The model under review builds one solid part; all positions refer to its coordinate system, in mm. A direction names the side the tool comes from. Give positions to 0.01 mm unless a question says otherwise; leave off trailing zeros. Loops run counter-clockwise (first coordinate to the right, second up) from the corner with the lowest first, then second, coordinate; pieces in that order, holes last. Notation, with made-up numbers: M 26.5,-9 L 50.5,-9 A17 ccw 50.5,8 Z; hole C 78,8 d9. An arc over 180 degrees is marked long. Write item = value, one per line. Start each with the question number.
1. For faces 1 (the face through (5, 41, -19)), 2 (the face through (4, 41, -29.25)), 3 (the face through (6, 41, -31)), list the 3-axis set-ups (+Z, -Z, +X, -X, +Y, -Y) from which the entire face can be reached by the end or side of a thin tool; tool diameter is ignored.
2. We need section B-B on z = -34. Give the boundary of the cut face in (x, y), then the cut area to 3 significant figures.
3. Wall thickness on line 1 along Z through (x, y) = (2.35, 71); line 2 along Z through (x, y) = (5, 39); line 3 along Z through (x, y) = (2.25, 71): over which ranges is each line inside the solid? List them lowest first. Write a range as from..to.
4. We need section D-D on y = 67.5. Give the boundary of the cut face in (x, z).
5. Draft analysis for pull direction Y (two halves, no side actions). For faces 4 (the face through (1, 14, -17)), 5 (the face through (1.479, 72.908, -15.601)), 6 (the face through (3, 40, -39)), 7 (the face through (2, 0, -13)), state which applies: pulls with the +Y half, pulls with the -Y half, needs draft (parallel to the pull), parting line crosses it, or undercut.
6. For pin 1 (5.5 mm diameter, centred on x = 3.5, y = 55.5, fed in from +Z); pin 2 (4.5 mm diameter, centred on y = 71, z = -15, fed in from +X); pin 3 (5 mm diameter, centred on x = 10.5, y = 38.5, fed in from +Z); pin 4 (2.5 mm diameter, centred on y = 14, z = -15, fed in from +X), all flat-tipped, find the tip position at first contact; note any pin that passes through.
7. We need section A-A on y = 14. Count the separate pieces of the cut face and the enclosed holes in it, then the cut area to 3 significant figures.
8. We need section C-C on x = 6. Give the boundary of the cut face in (y, z), then the cut area to 4 significant figures.
Autodesk Inventor part; units mm, degrees
ref_plane "YZ Plane" through (0, 0, 0) normal (1, 0, 0) x (0, 1, 0)
ref_plane "XZ Plane" through (0, 0, 0) normal (0, 1, 0) x (-1, 0, 0)
ref_plane "XY Plane" through (0, 0, 0) normal (0, 0, 1) x (1, 0, 0)
sketch "Sketch1" plane through (0, 0, 0) normal (1, 0, 0) x (0, 1, 0)
  line L0 (0, 0) -> (81, 0)
  line L1 (81, 0) -> (81, -50)
  line L2 (81, -50) -> (0, -50)
  line L3 (0, -50) -> (0, 0)
  circle A0 centre (71, -15) radius 2
  circle A1 centre (71, -34) radius 2
  circle A2 centre (14, -15) radius 2
  circle A3 centre (14, -34) radius 2
  dimension "d0" = 81
  dimension "d1" = 50
  dimension "d2" = 4
  dimension "d3" = 15
  dimension "d4" = 4
  dimension "d5" = 16
  dimension "d6" = 4
  dimension "d7" = 15
  dimension "d8" = 4
  dimension "d9" = 57
  dimension "d11" = 10
  dimension "d12" = 57
  dimension "d13" = 10
extrude "Extrusion1" add sketch "Sketch1" along normal blind 3
sketch "Sketch5" plane through (0, 81, 0) normal (0, 1, 0) x (1, 0, 0)
  circle A0 centre (7, 25) radius 4
  line L0 (0, 0) -> (3, 0)
  line L1 (3, 50) -> (3, 0)
  dimension "d26" = 8
  dimension "d27" = 25
  dimension "d28" = 4
extrude "Extrusion3" add sketch "Sketch5" against normal blind 81
sketch "Sketch9" plane through (7, 81, -25) normal (0, 1, 0) x (1, 0, 0)
  line L0 (-4, 0) -> (-4, -25)
  line L1 (-4, -6) -> (6, -6)
  line L2 (6, -6) -> (6, 6)
  line L3 (6, 6) -> (-4, 6)
  line L4 (-4, 6) -> (-4, -6)
  line L5 (-7, -25) -> (-4, -25)
  dimension "d42" = 10
  dimension "d43" = 12
  dimension "d44" = 19
extrude "Extrusion6" add sketch "Sketch9" against normal blind 81
sketch "Sketch10" plane through (0, 81, 0) normal (0, 1, 0) x (1, 0, 0)
  line L0 (3, 19) -> (13, 19)
  line L1 (13, 19) -> (13, 31)
  line L2 (7, 29.25) -> (0, 29.25)
  line L3 (0, 50) -> (0, 0)
  line L4 (7, 20.75) -> (0, 20.75)
  arc A0 (7, 20.75) -> (7, 29.25) centre (7, 25) ccw
  arc A1 (7, 20.75) -> (7, 29.25) centre (7, 25) ccw
  arc A2 (7, 20.75) -> (7, 29.25) centre (7, 25) ccw
  dimension "d55" = 4.25
  dimension "d56" = 4.25
  dimension "d57" = 4.25
extrude "Extrusion8" cut sketch "Sketch10" against normal blind 81
fillet "Fillet4" radius 4 2 edges at (3, 40.5, 0) (3, 40.5, -50)
fillet "Fillet5" radius 1 2 edges at (3, 40.5, -19) (3, 40.5, -31)
fillet "Fillet6" radius 6 4 edges at (13, 81, -25) (13, 0, -25) (13, 40.5, -19) (13, 40.5, -31)
Final values:
q1.face_1 = +Z, +X, +Y, -Y
q1.face_2 = -X, +Y, -Y
q1.face_3 = -Z, +X, +Y, -Y
q2.outline = M 0,0 L 3,0 L 3,12 L 0,12 Z; M 0,16 L 3,16 L 3,69 L 0,69 Z; M 0,73 L 3,73 L 3,81 L 0,81 Z
q2.area = 219 mm²
q3.line_1 = -48.31..-36, -32..-29.25, -20.75..-17, -13..-1.69
q3.line_2 = -31..-29.25, -20.75..-19
q3.line_3 = -48.46..-36, -32..-29.25, -20.75..-17, -13..-1.54
q4.outline = M 0,-50 A4 ccw 3,-46.13 L 3,-32 A1 cw 4,-31 L 7,-31 A6 ccw 7,-19 L 4,-19 A1 cw 3,-18 L 3,-3.87 A4 ccw 0,0 L 0,-20.75 L 7,-20.75 A4.25 cw 7,-29.25 L 0,-29.25 Z
q5.face_4 = undercut
q5.face_5 = undercut
q5.face_6 = needs draft
q5.face_7 = pulls with the -Y half
q6.pin_1 = -0.28
q6.pin_2 = 3
q6.pin_3 = -19.08
q6.pin_4 = through
q7.separate_pieces = 3
q7.enclosed_holes = 0
q7.area = 137 mm²
q8.outline = M 0,-31 L 81,-31 L 81,-29.25 L 0,-29.25 Z; M 0,-20.75 L 81,-20.75 L 81,-19 L 0,-19 Z
q8.area = 283.5 mm²
